Input: dimensioned drawing with shaded views. Units: mm. Origin: part minimum x, y, z. Round coordinates to 2 decimals unless told otherwise and drop trailing zeros. Order: outer loops, then holes, each group sorted by start corner. A loop starts at its lowest first (then second) coordinate and runs counter-clockwise, first axis right, second up.
Item 1: Cut plane B-B on y = 24.8. Output: boundary loops of the cut face in (x, z), then the cut area to 3 significant figures.
Item 2: First-contact query: pin 1 (2.5 mm diameter, centred on x = 52.5, y = 24.8, fed in from +Z). Flat tip, straight axial feed; report the tip coordinate or a pass-through.
Item 3: Cut plane D-D on y = 33. Output: boundary loops of the cut face in (x, z), then the cut area to 3 significant figures.
Item 4: Line query: L1, parallel to X at y = 26, z = 1.55; L2, parallel to Y at x = 30, z = 1.25; L3, parallel to X at y = 27.5, z = 1.55. Output: solid intervals per line, ascending.
Item 5: Cut plane C-C on z = 1.55. Output: boundary loops of the cut face in (x, y), then the cut area to 3 significant figures.
Item 6: Cut plane A-A on x = 30. Output: boundary loops of the cut face in (y, z), then the cut area to 3 significant figures.
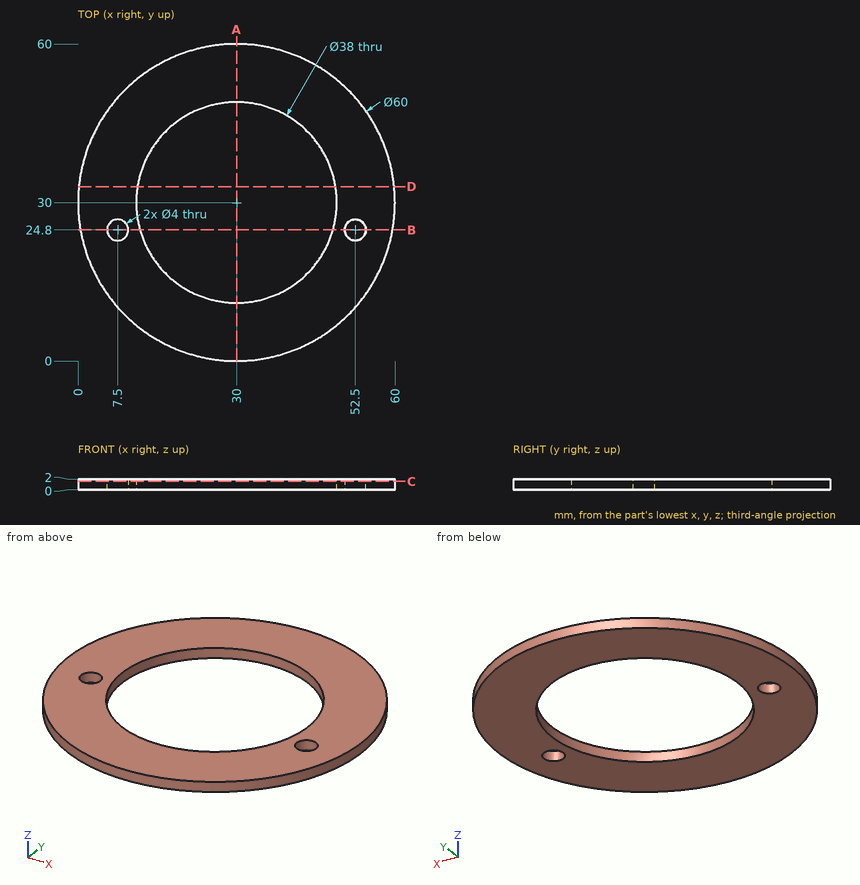
From the geometry:
1. outline: (0.45, 0) - (5.5, 0) - (5.5, 2) - (0.45, 2) - close; (9.5, 0) - (11.73, 0) - (11.73, 2) - (9.5, 2) - close; (48.27, 0) - (50.5, 0) - (50.5, 2) - (48.27, 2) - close; (54.5, 0) - (59.55, 0) - (59.55, 2) - (54.5, 2) - close
1. area: 29.1 mm2
2. pin 1: passes through
3. outline: (0.15, 0) - (11.24, 0) - (11.24, 2) - (0.15, 2) - close; (48.76, 0) - (59.85, 0) - (59.85, 2) - (48.76, 2) - close
3. area: 44.4 mm2
4. L1: x = 0.27 to 5.9, 9.1 to 11.43, 48.57 to 50.9, 54.1 to 59.73
4. L2: y = 0 to 11, 49 to 60
4. L3: x = 0.1 to 11.17, 48.83 to 59.9
5. outline: circle Ø60 at (30, 30); hole circle Ø4 at (7.5, 24.8); hole circle Ø38 at (30, 30); hole circle Ø4 at (52.5, 24.8)
5. area: 1,670 mm2
6. outline: (0, 0) - (11, 0) - (11, 2) - (0, 2) - close; (49, 0) - (60, 0) - (60, 2) - (49, 2) - close
6. area: 44.0 mm2
